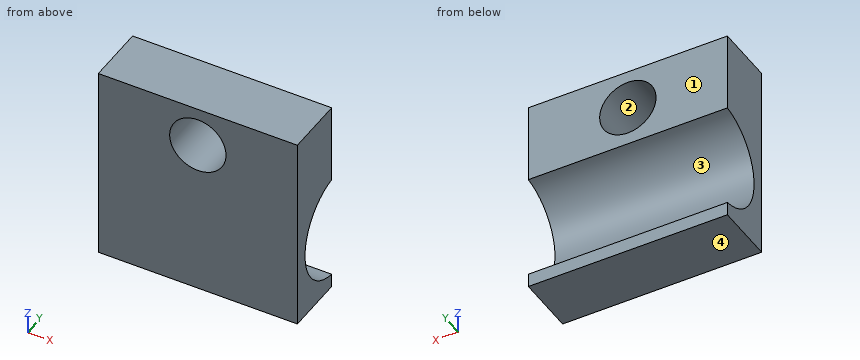
```python
from build123d import *

# Parameters (mm, degrees)
SKETCH1_W           = 15
SKETCH1_H           = 15
SKETCH1_R           = 2.125
BOSS_EXTRUDE1_DEPTH = 4.5
CUT_EXTRUDE1_REACH  = 23.685
SKETCH2_R           = 4


with BuildPart() as part:
    # Sketch1 → Boss-Extrude1 (new body)
    with BuildSketch(Plane(origin=(0, 0, 0), x_dir=(1, 0, 0), z_dir=(0, 1, 0))):
        with Locations((-7.5, 7.5)):
            Rectangle(SKETCH1_W, SKETCH1_H)
        with Locations(Location((-7.5, 3, 0), (0, 0, 270))):
            Circle(SKETCH1_R, mode=Mode.SUBTRACT)
    extrude(amount=BOSS_EXTRUDE1_DEPTH)

    # Sketch2 → Cut-Extrude1 (cut, up to next)
    with BuildSketch(Plane(origin=(0, 0, 0), x_dir=(0, 0, -1), z_dir=(1, 0, 0)), mode=Mode.PRIVATE) as cut_extrude1_sk1:
        with Locations((10, 5)):
            Circle(SKETCH2_R)
    cut_extrude1_tool1 = extrude(cut_extrude1_sk1.sketch, amount=-CUT_EXTRUDE1_REACH, mode=Mode.PRIVATE) & part.part
    add(cut_extrude1_tool1.solids().sort_by_distance((0, 5, -10))[0], mode=Mode.SUBTRACT)


solid = part.part
```
Here's how the part is built. I have some questions about the finished solid (model axes, mm). Face numbers are marked on the shaded views. Round coordinates to 2 decimals unless told otherwise and drop trailing zeros. Write each loop counter-clockwise with the first axis right and the second up, starting at its lowest first coordinate (ties: lowest second). Pieces come first, ordered by that corner, then holes.
Q1. Please list where these lines run through material, in increasing order: probe 1 along X at (y, z) = (2.05, -3) (3 decimals); probe 2 along Z at (x, y) = (-6.5, 2.6) (3 decimals); probe 3 along Z at (x, y) = (-6.5, 1.5) (1 decimal).
Q2. If we section it at B-B on y = 3.55: Write out the boundary of the cut face in (x, z) (3 decimals), plus the area to 3 significant figures.
Q3. If we mould it in two halves opening along Z, with no side actions, what happens to the marked faces 1, 2, 3 and 4? For each: +Z half, -Z half, draft (parallel to the pull), parting line (faces both ways), or undercut.
Q4. If we section it at A-A on x = -7.5: Write out the boundary of the cut face in (y, z) (3 decimals).
Q5. If we section it at D-D on x = -13: Write out the boundary of the cut face in (y, z).
Q6. If we section it at C-C on z = -3: Write out the boundary of the cut face in (x, y) (3 decimals).
Answer below:
1. probe 1: x = -15 to -9.625, -5.375 to 0
1. probe 2: z = -15 to -13.2, -6.8 to -4.875, -1.125 to 0
1. probe 3: z = -15 to -11.9, -8.1 to -4.9, -1.1 to 0
2. outline: (-15, -15) - (0, -15) - (0, -13.728) - (-15, -13.728) - close; (-15, -6.272) - (0, -6.272) - (0, 0) - (-15, 0) - close; hole circle Ø4.25 at (-7.5, -3)
2. area: 99.0 mm2
3. face 1: draft
3. face 2: undercut
3. face 3: undercut
3. face 4: -Z half
4. outline: (0, -15) - (4.5, -15) - (4.5, -13.969) arc R4 cw to (4.5, -6.031) - (4.5, -5.125) - (0, -5.125) - close; (0, -0.875) - (4.5, -0.875) - (4.5, 0) - (0, 0) - close
5. outline: (0, -15) - (4.5, -15) - (4.5, -13.97) arc R4 cw to (4.5, -6.03) - (4.5, 0) - (0, 0) - close
6. outline: (-15, 0) - (-9.625, 0) - (-9.625, 4.5) - (-15, 4.5) - close; (-5.375, 0) - (0, 0) - (0, 4.5) - (-5.375, 4.5) - close
